Geometry: final body of the model. Coordinates: model frame, mm. Face numbers are marked on the shaded views. Round coordinates to 2 decimals unless told otherwise and drop trailing zeros. Loops run counter-clockwise (first coordinate to the right, second up) from the corner with the lowest first, then second, coordinate; pieces in that order, holes last. Notation, with made-up numbers: (40.5, 89) - (51.5, 89) arc R31 ccw to (51.5, 117) - close; hole circle Ø11 at (-1.5, 44). An arc over 180 degrees is marked (long way). Answer as CSV lines item,"result".
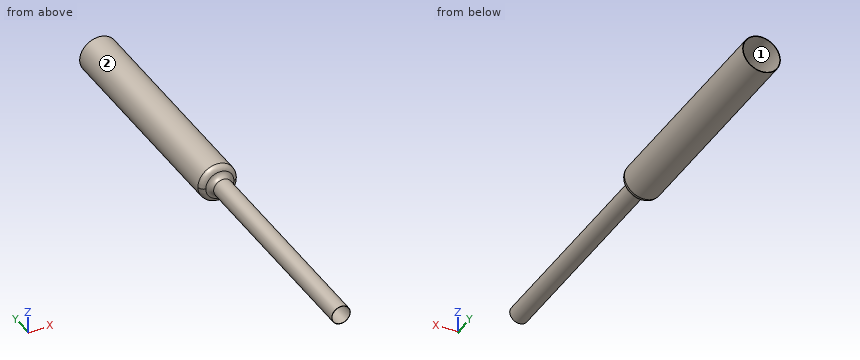
Autodesk Inventor part; units mm, degrees
ref_plane "YZ Plane" through (0, 0, 0) normal (1, 0, 0) x (0, 1, 0)
ref_plane "XZ Plane" through (0, 0, 0) normal (0, 1, 0) x (-1, 0, 0)
ref_plane "XY Plane" through (0, 0, 0) normal (0, 0, 1) x (1, 0, 0)
sketch "Sketch1" plane through (0, 0, 0) normal (0, 1, 0) x (-1, 0, 0)
  circle A0 centre (0, 0) radius 12.5
  circle A1 centre (0, 0) radius 12.192
  dimension "d0" = 25
  dimension "d1" = 24.384
extrude "Extrusion1" add sketch "Sketch1" along normal blind 304.8
sketch "Sketch2" plane through (0, 304.8, 0) normal (0, 1, 0) x (1, 0, 0)
  circle A0 centre (0, 0) radius 24.765
  circle A1 centre (0, 0) radius 25.4
  dimension "d4" = 50.8
  dimension "d5" = 49.53
extrude "Extrusion2" add sketch "Sketch2" along normal blind 304.8
sketch "Sketch3" plane through (0, 304.8, 0) normal (0, -1, 0) x (1, 0, 0)
  circle A0 centre (0, 0) radius 25.4
  circle A1 centre (0, 0) radius 12.192
  dimension "d8" = 50.8
  dimension "d12" = 24.384
extrude "Extrusion3" add sketch "Sketch3" against normal blind 1.27
fillet "Fillet1" radius 7.874 3 edges at (12.5, 304.8, 0) (-24.765, 306.07, 0) (-25.4, 304.8, 0)
fillet "Fillet2" radius 7.874 1 edges at (-12.192, 306.07, 0)
properties part number "still pipe standin" material "Stainless Steel, Austenitic"
(1) Section A-A (y = 188). Output: boundary loops of the cut face in (x, z).
Findings below:
outline,"circle Ø25 at (0, 0); hole circle Ø24.38 at (0, 0)"
(2) Section B-B (y = 519.5). Output: boundary loops of the cut face in (x, z) (3 decimals), and give its area (3 significant figures).
Findings below:
outline,"circle Ø50.8 at (0, 0); hole circle Ø49.53 at (0, 0)"
area,"100 mm2"
(3) Draft query along X for the marked faces 1 and 2. Return one class per face: pulls with the +X half, pulls with the -X half, needs draft (parallel to the pull), parting line crosses it, or undercut.
Findings below:
face 1,"undercut"
face 2,"parting line crosses it"
(4) Pin query (flat end, axial travel): P1, Ø4, axis at x = 9, y = 151, coming from the +Z side; P2, Ø10, axis at y = 546, z = 4, coming from the -X side; P3, Ø6, axis at x = 2.5, z = 7, coming from the +Y side; P4, Ø2, axis at y = 280, z = -9, coming from the +X side. Return the tip coordinate at first contact, or that it passes through.
Findings below:
P1,"z = 10.36"
P2,"x = -25.4"
P3,"through"
P4,"x = 9.6"
(5) Material intervals for line 1 along Z through (x, y) = (0, 78); line 2 along Z through (x, y) = (0.5, 381.5); line 3 along X through (y, z) = (414.5, 2), sorted ascending.
Findings below:
line 1,"-12.5 to -12.19, 12.19 to 12.5"
line 2,"-25.4 to -24.76, 24.76 to 25.4"
line 3,"-25.32 to -24.68, 24.68 to 25.32"
